CAD build for the part. Positions are in the model's coordinates, mm. Round coordinates to 2 decimals unless told otherwise and drop trailing zeros. Loops run counter-clockwise (first coordinate to the right, second up) from the corner with the lowest first, then second, coordinate; pieces in that order, holes last.
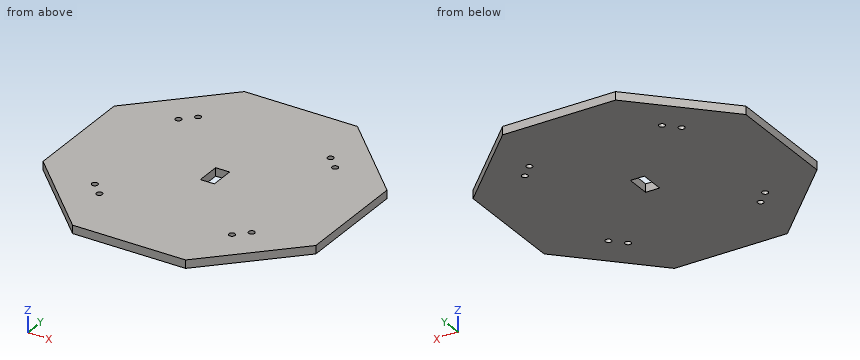
```python
from build123d import *

# Parameters (mm, degrees)
F1_DEPTH = 3.048
F3_D     = 2.2606
F4_W     = 5.1865465939
F4_H     = 9.0437950566
F5_DEPTH = 25.4


with BuildPart() as f1:
    # F0 (on Top) → F1 (new body)
    with BuildSketch(Plane.XY):
        Polygon((21.0420489686, 50.8), (-21.0420489686, 50.8), (-50.8, 21.0420489686), (-50.8, -21.0420489686), (-21.0420489686, -50.8), (21.0420489686, -50.8), (50.8, -21.0420489686), (50.8, 21.0420489686), align=None)
    extrude(amount=F1_DEPTH)

    # F3 (through all)
    with Locations(Plane.XY.offset(3.048)):
        with Locations((-24.6957043329, 29.1858323935), (-29.1858323935, 24.6957043329), (-29.1858323935, -24.6957043329), (-24.6957043329, -29.1858323935), (24.6957043329, -29.1858323935), (29.1858323935, -24.6957043329), (29.1858323935, 24.6957043329), (24.6957043329, 29.1858323935)):
            Hole(F3_D / 2)

    # F4 (on face) → F5 (cut)
    with BuildSketch(Plane.XY.offset(3.048)):
        Rectangle(F4_W, F4_H)
    extrude(amount=-F5_DEPTH, mode=Mode.SUBTRACT)


solid = f1.part
```
Item 1: Cut at A-A, the plane y = 0. Give the cut face in (x, z).
Answers follow:
outline: (-50.8, 0) - (-2.59, 0) - (-2.59, 3.05) - (-50.8, 3.05) - close; (2.59, 0) - (50.8, 0) - (50.8, 3.05) - (2.59, 3.05) - close
Item 2: Cut at B-B, the plane z = 1.25. State how many separate pieces and enclosed holes the cut face has, plus the area to 3 significant figures.
Answers follow:
separate pieces: 1
enclosed holes: 9
area: 8,470 mm2
Item 3: Flat gauge pins, fed straight in: P1, Ø2.5, axis at x = -29.19, y = -24.7, coming from the +Z side; P2, Ø2, axis at x = -24.7, y = 29.19, coming from the -Z side. Where does each tip first touch, or does it go through?
Answers follow:
P1: stops at z = 3.05
P2: passes through
Item 4: Cut at D-D, the plane y = 44.5. Give the cut face in (x, z).
Answers follow:
outline: (-27.34, 0) - (27.34, 0) - (27.34, 3.05) - (-27.34, 3.05) - close
Item 5: Probe line 1 (X direction, y = 30, z = 1.55); line 2 (Y direction, x = -24, z = 2.55) (3 decimals); line 3 (X direction, y = 3, z = 1.4). List the from-to ranges inside material, lowest first.
Answers follow:
line 1: x = -41.84 to -25.48, -23.91 to 23.91, 25.48 to 41.84
line 2: y = -47.842 to -30.077, -28.295 to 28.295, 30.077 to 47.842
line 3: x = -50.8 to -2.59, 2.59 to 50.8
Item 6: Cut at C-C, the plane y = -39. Give the cut face in (x, z).
Answers follow:
outline: (-32.84, 0) - (32.84, 0) - (32.84, 3.05) - (-32.84, 3.05) - close
